```python
from build123d import *

# Parameters (mm, degrees)
F0_R          = 20
F1_DEPTH      = 8
F2_R          = 18
F2_W          = 30
F2_H          = 5
F3_DEPTH      = 2
F6_END_RADIUS = 18
F5_W          = 16
F5_H          = 8
F6_REACH      = 57.88954382
F7_D          = 3.5
F7_DEPTH      = 8
F7_TIP        = 1.0515060833
F8_R          = 1


with BuildPart() as f1:
    # F0 (on Top) → F1 (new body)
    with BuildSketch(Plane.XY):
        Circle(F0_R)
    extrude(amount=F1_DEPTH)

    # F2 (on face) → F3 (cut)
    with BuildSketch(Plane.XY.offset(8)):
        Circle(F2_R)
        Rectangle(F2_W, F2_H, mode=Mode.SUBTRACT)
    extrude(amount=-F3_DEPTH, mode=Mode.SUBTRACT)

    f6_end = (Plane.XY.offset(7) * Cylinder(F6_END_RADIUS, 230.0419424967, mode=Mode.PRIVATE)).faces().sort_by_distance((-18, 0, 7))[0]
    # F5 (on offset) → F6 (join, up to the whole of a round face its end follows)
    with BuildSketch(Plane.XZ.offset(20)):
        with Locations((0, 4)):
            Rectangle(F5_W, F5_H)
    f6_long = extrude(amount=-F6_REACH, mode=Mode.PRIVATE)
    add(split(f6_long, bisect_by=f6_end, keep=Keep.ALL, mode=Mode.PRIVATE).solids().sort_by_distance((0, -20, 4))[0])

    # F7
    with Locations(Plane.XZ.offset(20)):
        with Locations((4, 4), (-4, 4)):
            Hole(F7_D / 2, depth=F7_DEPTH)
            with Locations((0, 0, -(F7_DEPTH + F7_TIP / 2))):  # 118° drill point
                Cone(0, F7_D / 2, F7_TIP, mode=Mode.SUBTRACT)

    # F8
    f8_edges = [f1.edges().sort_by_distance(p)[0] for p in [
        (8, -18.330303, 4),
        (-8, -18.330303, 4),
    ]]
    fillet(f8_edges, radius=F8_R)


solid = f1.part
```
For this review, take the finished solid that the model builds, in its own axes (mm). A direction names the side the tool comes from. Give positions to 0.01 mm unless a question says otherwise; leave off trailing zeros. Write each loop counter-clockwise with the first axis right and the second up, starting at its lowest first coordinate (ties: lowest second). Pieces come first, ordered by that corner, then holes.
Item 1: Take a section at C-C (x = 0). Give the boundary of the cut face in (y, z).
Item 2: The part is to be moulded in two halves that separate along Z. For faces 4 (the face through (4.29, -11.13, 4.09)), 5 (the face through (-8, -19.5, 3.9)), 6 (the face through (0, 0, 0)), say which applies: +Z half, -Z half, draft (parallel to the pull), parting line (faces both ways), or undercut.
Item 3: Take a section at D-D (z = 1.75). Give the boundary of the cut face in (x, y).
Item 4: Wall thickness on probe 1 along Y at (x, z) = (0, 6.55); probe 2 along X at (y, z) = (0, 7.4); probe 3 along Z at (x, y) = (4, -14): over which ranges is each line inside the solid? List them lowest first.
Item 5: Insertion check: P1, Ø4, axis at x = -4.5, y = -3, coming from the +Z side; P2, Ø8, axis at x = 8.5, y = -9.5, coming from the +Z side; P3, Ø4, axis at y = -2.5, z = 1, coming from the -X side; P4, Ø1, axis at x = -2.5, z = 6, coming from the +Y side. Each pin has a flat end and moves straight along its axis. Give the tip position at first contact, or say it passes through.
Item 6: Take a section at B-B (y = -16). Give the boundary of the cut face in (x, z).
Item 7: Take a section at A-A (y = 0). Give the boundary of the cut face in (x, z), and give its area (3 significant figures).
Item 8: Machinability: for faces 1 (the face through (5.39, -15.94, 2.94)), 2 (the face through (8, -19.5, 3.9)), 3 (the face through (-2.343, 17.847, 7.014)), which of the approach directions +Z, -Z, +X, -X, +Y, -Y give a long, thin tool a straight path to every point of the face, cutting with its end or side? Answer none if there is none.
Established:
1. outline: (-20, 0) - (20, 0) - (20, 8) - (18, 8) - (18, 6) - (2.5, 6) - (2.5, 8) - (-2.5, 8) - (-2.5, 6) - (-18, 6) - (-18, 8) - (-20, 8) - close
2. face 4: undercut
2. face 5: draft
2. face 6: -Z half
3. outline: (-8.57, -18.07) arc R1 cw to (-8, -18.97) - (-8, -20) - (8, -20) - (8, -18.97) arc R1 cw to (8.57, -18.07) arc R20 ccw (long way) to start
4. probe 1: y = -20 to -18, -2.5 to 2.5, 18 to 20
4. probe 2: x = -20 to -18, -15 to 15, 18 to 20
4. probe 3: z = 0 to 2.25, 5.75 to 6
5. P1: stops at z = 8
5. P2: stops at z = 6
5. P3: stops at x = -19.99
5. P4: stops at y = 19.9
6. outline: (-12, 0) - (12, 0) - (12, 8) - (8.25, 8) - (8.25, 6) - (-8.25, 6) - (-8.25, 8) - (-12, 8) - close; hole circle Ø3.5 at (-4, 4); hole circle Ø3.5 at (4, 4)
7. outline: (-20, 0) - (20, 0) - (20, 8) - (18, 8) - (18, 6) - (15, 6) - (15, 8) - (-15, 8) - (-15, 6) - (-18, 6) - (-18, 8) - (-20, 8) - close
7. area: 308 mm2
8. face 1: -Y
8. face 2: +Z, -Z, +X, -Y
8. face 3: +Z
